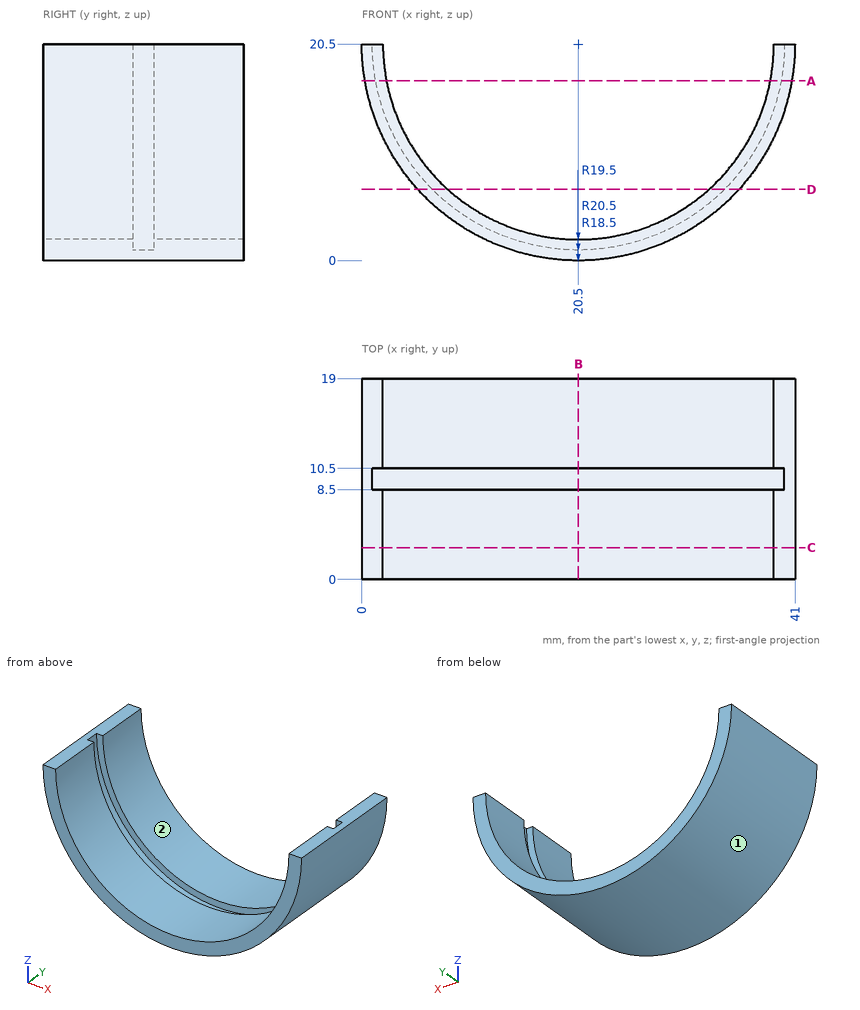
Answer from the drawing. Dimensions are ordinates in mm from the lowest x, y and z of the part. Round coordinates to 2 decimals unless told otherwise and drop trailing zeros. Write each loop counter-clockwise with the first axis right and the second up, starting at its lowest first coordinate (ties: lowest second). Pieces come first, ordered by that corner, then holes. Notation, with made-up numbers: (85.25, -5) - (96.25, -5) arc R34 cw to (96.25, 34) - close; hole circle Ø11 at (78, 16.25). An arc over 180 degrees is marked (long way). Use a Markdown table: item, result.
(1) Each of these flat-tipped pins is pushed along its axis until it touches: pin 1 Ø4 at (y, z) = (12.5, 15.5) entering from -X; pin 2 Ø4 at (x, y) = (19.5, 8) entering from -Z; pin 3 Ø8 at (x, y) = (8.5, 16) entering from +Z. Where does it stop, or does it pass through?
Reported:
| item | result |
|---|---|
| pin 1 | x = 0.22 |
| pin 2 | z = 0 |
| pin 3 | z = 11.21 |
(2) The part is cut by section C-C (y = 3). Write down the section's boundary in (x, z), then the cut area to 3 significant figures.
Reported:
| item | result |
|---|---|
| outline | (0, 20.5) arc R20.5 ccw to (41, 20.5) - (39, 20.5) arc R18.5 cw to (2, 20.5) - close |
| area | 123 mm2 |
(3) The mould has two halves that part along X. Classify the marked faces 1 and 2: released by +X, released by -X, zero draft, split by the parting line, or undercut.
Reported:
| item | result |
|---|---|
| face 1 | split by the parting line |
| face 2 | undercut |
(4) The part is cut by section A-A (z = 17). Write down the section's boundary in (x, y).
Reported:
| item | result |
|---|---|
| outline | (0.3, 0) - (2.33, 0) - (2.33, 8.5) - (1.32, 8.5) - (1.32, 10.5) - (2.33, 10.5) - (2.33, 19) - (0.3, 19) - close; (38.67, 0) - (40.7, 0) - (40.7, 19) - (38.67, 19) - (38.67, 10.5) - (39.68, 10.5) - (39.68, 8.5) - (38.67, 8.5) - close |
(5) Straight lines are drawn through the part: line 1 along Y through (x, z) = (2.5, 16); line 2 along X through (y, z) = (6, 5.5); line 3 along X through (y, z) = (18, 18.75). For each, find the intervals that lie inside material, in ascending order. Write a range as [from, to].
Reported:
| item | result |
|---|---|
| line 1 | [0, 8.5], [10.5, 19] |
| line 2 | [6.53, 9.67], [31.33, 34.47] |
| line 3 | [0.07, 2.08], [38.92, 40.93] |
(6) The part is cut by section B-B (x = 20.5). Write down the section's boundary in (y, z).
Reported:
| item | result |
|---|---|
| outline | (0, 0) - (19, 0) - (19, 2) - (10.5, 2) - (10.5, 1) - (8.5, 1) - (8.5, 2) - (0, 2) - close |
(7) The part is cut by section D-D (z = 6.75). Write down the section's boundary in (x, y).
Reported:
| item | result |
|---|---|
| outline | (5.3, 0) - (8.12, 0) - (8.12, 8.5) - (6.67, 8.5) - (6.67, 10.5) - (8.12, 10.5) - (8.12, 19) - (5.3, 19) - close; (32.88, 0) - (35.7, 0) - (35.7, 19) - (32.88, 19) - (32.88, 10.5) - (34.33, 10.5) - (34.33, 8.5) - (32.88, 8.5) - close |
